Build history of the part. All positions in model axes, mm. Face numbers are marked on the shaded views. A direction names the side the tool comes from. Coordinates: 2 decimals unless noted, no trailing zeros. Write each loop counter-clockwise with the first axis right and the second up, starting at its lowest first coordinate (ties: lowest second). Pieces come first, ordered by that corner, then holes.
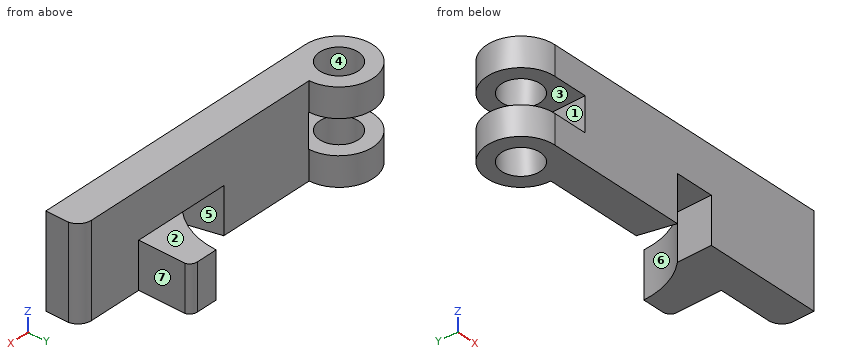
from build123d import *

# Parameters (mm, degrees)
F0_R     = 12.7
F1_DEPTH = 60.325
F2_DEPTH = 30.1625
F3_W     = 31.937063
F3_H     = 22.3266
F3_W_2   = 22.687722
F4_DEPTH = 56.743083
F6_DEPTH = 30.1625


with BuildPart() as f1:
    # F0 (on Top) → F1 (new body)
    with BuildSketch(Plane.XY):
        with BuildLine():
            Line((85.852, 0), (22.352, 0))
            ThreePointArc((22.352, 0), (-15.805251, 15.805251), (0, -22.352))
            Line((0, -22.352), (91.8464, -22.352))
            Line((91.8464, -22.352), (85.852, 0))
        make_face()
        Circle(F0_R, mode=Mode.SUBTRACT)
        Polygon((117.2464, 0), (85.852, 0), (91.8464, -22.352), (117.2464, -22.352), align=None)
        with BuildLine():
            Line((150.0886, 0), (117.2464, 0))
            Line((117.2464, 0), (117.2464, -22.352))
            Line((117.2464, -22.352), (194.2084, -22.352))
            Line((194.2084, -22.352), (194.2084, -7.573048))
            ThreePointArc((194.2084, -7.573048), (191.161905, -2.150228), (185.325414, 0))
            Line((185.325414, 0), (162.975117, 0))
            Line((162.975117, 0), (150.0886, 0))
        make_face()
    extrude(amount=F1_DEPTH)

    # F0 (on Top) → F2 (join)
    with BuildSketch(Plane.XY):
        with BuildLine():
            Line((85.852, 0), (22.352, 0))
            ThreePointArc((22.352, 0), (-15.805251, 15.805251), (0, -22.352))
            Line((0, -22.352), (91.8464, -22.352))
            Line((91.8464, -22.352), (85.852, 0))
        make_face()
        Circle(F0_R, mode=Mode.SUBTRACT)
        Polygon((117.2464, 0), (85.852, 0), (91.8464, -22.352), (117.2464, -22.352), align=None)
        with BuildLine():
            Line((150.0886, 0), (117.2464, 0))
            Line((117.2464, 0), (117.2464, -22.352))
            Line((117.2464, -22.352), (194.2084, -22.352))
            Line((194.2084, -22.352), (194.2084, -7.573048))
            ThreePointArc((194.2084, -7.573048), (191.161905, -2.150228), (185.325414, 0))
            Line((185.325414, 0), (162.975117, 0))
            Line((162.975117, 0), (150.0886, 0))
        make_face()
        with BuildLine():
            ThreePointArc((131.0386, 34.390083), (127.389769, 15.892719), (117.2464, 0))
            Line((117.2464, 0), (150.0886, 0))
            Line((150.0886, 0), (150.0886, 30.665313))
            ThreePointArc((150.0886, 30.665313), (148.268569, 33.353038), (145.192709, 34.390083))
            Line((145.192709, 34.390083), (131.0386, 34.390083))
        make_face()
    extrude(amount=F2_DEPTH)

    # F3 (on face) → F4 (cut, through all)
    with BuildSketch(Plane.XZ.offset(22.352)):
        with Locations((-15.968531, 30.1625)):
            Rectangle(F3_W, F3_H)
        with Locations((11.343861, 30.1625)):
            Rectangle(F3_W_2, F3_H)
    extrude(amount=-F4_DEPTH, mode=Mode.SUBTRACT)

    # F5 (on face) → F6 (cut)
    with BuildSketch(Plane(origin=(0, 0, 0), x_dir=(1, 0, 0), z_dir=(0, 0, -1))):
        Polygon((86.316593, 0), (117.2464, 0), (117.2464, 22.352), (91.8464, 22.352), align=None)
    extrude(amount=-F6_DEPTH, mode=Mode.SUBTRACT)


solid = f1.part
(1) 3-axis set-ups, long thin cutter, end or side, ignore diameter. For the marked faces 5, 6 and 7: which of +Z, -Z, +X, -X, +Y, -Y reach the whole face in a straight line?
(2) Slice it at D-D, the plane y = -18. List the corners of the cut face in (x, z) (1 decimal), and give its area (3 significant figures).
(3) Probe L1, parallel to Y at x = 0, z = 9.75; L2, parallel to Z at x = -8, y = 16 (3 decimals); L3, parallel to Y at x = 32, z = 3. List the from-to ranges inside material, lowest first.
(4) Flat gauge pins, fed straight in: P1, Ø1.5, axis at y = 3.5, z = 23.5, coming from the -X side; P2, Ø11, axis at x = 102, y = -10.5, coming from the -Z side; P3, Ø9, axis at y = 16, z = 15, coming from the +X side. Where does each tip first touch, or does it go through?
(5) Slice it at A-A, the plane y = 10.5. List the corners of the cut face in (x, z) (1 decimal).
(6) Slice it at B-B, the plane z = 43.5. List the corners of the cut face in (x, y), and give its area (3 significant figures).
(7) Two-plate mould, pull along Z, no slides. Class the marked faces 1, 2, 3 and 4: pulls with the +Z half, pulls with the -Z half, needs draft (parallel to the pull), parting line crosses it, or undercut.
(8) Slice it at C-C, the plane y = -3. List the corners of the cut face in (x, z) (1 decimal), and give its area (3 significant figures).
Results:
1. face 5: -Z, +Y
1. face 6: +Z, -Z, +Y
1. face 7: +Z, -Z, +X, +Y
2. outline: (-13.3, 0) - (90.8, 0) - (90.8, 30.2) - (117.2, 30.2) - (117.2, 0) - (194.2, 0) - (194.2, 60.3) - (-13.3, 60.3) - (-13.3, 41.3) - (22.7, 41.3) - (22.7, 19) - (-13.3, 19) - close
2. area: 10,900 mm2
3. L1: y = -22.35 to -12.7, 12.7 to 22.35
3. L2: z = 0 to 18.999, 41.326 to 60.325
3. L3: y = -22.35 to 0
4. P1: stops at x = 119.65
4. P2: stops at z = 30.16
4. P3: stops at x = 150.09
5. outline: (-19.7, 0) - (-7.1, 0) - (-7.1, 19) - (-19.7, 19) - close; (-19.7, 41.3) - (-7.1, 41.3) - (-7.1, 60.3) - (-19.7, 60.3) - close; (7.1, 0) - (19.7, 0) - (19.7, 19) - (7.1, 19) - close; (7.1, 41.3) - (19.7, 41.3) - (19.7, 60.3) - (7.1, 60.3) - close; (124.9, 0) - (150.1, 0) - (150.1, 30.2) - (124.9, 30.2) - close
6. outline: (0, -22.35) - (194.21, -22.35) - (194.21, -7.57) arc R9 ccw to (185.33, 0) - (22.35, 0) arc R22.35 ccw (long way) to start; hole circle Ø25.4 at (0, 0)
6. area: 4,990 mm2
7. face 1: undercut
7. face 2: pulls with the +Z half
7. face 3: undercut
7. face 4: needs draft
8. outline: (-22.1, 0) - (-12.3, 0) - (-12.3, 19) - (-22.1, 19) - close; (-22.1, 41.3) - (-12.3, 41.3) - (-12.3, 60.3) - (-22.1, 60.3) - close; (12.3, 0) - (87.1, 0) - (87.1, 30.2) - (117.2, 30.2) - (117.2, 0) - (192, 0) - (192, 60.3) - (12.3, 60.3) - (12.3, 41.3) - (22.7, 41.3) - (22.7, 19) - (12.3, 19) - close
8. area: 10,100 mm2
